The drawing under review shows one solid part. Ordinate dimensions are in mm from its lowest x, y, z. A direction names the side the tool comes from. Round coordinates to 2 decimals unless told otherwise and drop trailing zeros. Loops run counter-clockwise (first coordinate to the right, second up) from the corner with the lowest first, then second, coordinate; pieces in that order, holes last. Notation, with made-up numbers: (48.5, 16.25) -> (101.5, 16.25) arc R26 ccw to (101.5, 37.25) -> close; hole circle Ø4 at (-28, 15). An arc over 180 degrees is marked (long way). Use a Markdown table: item, result. Add a question column.
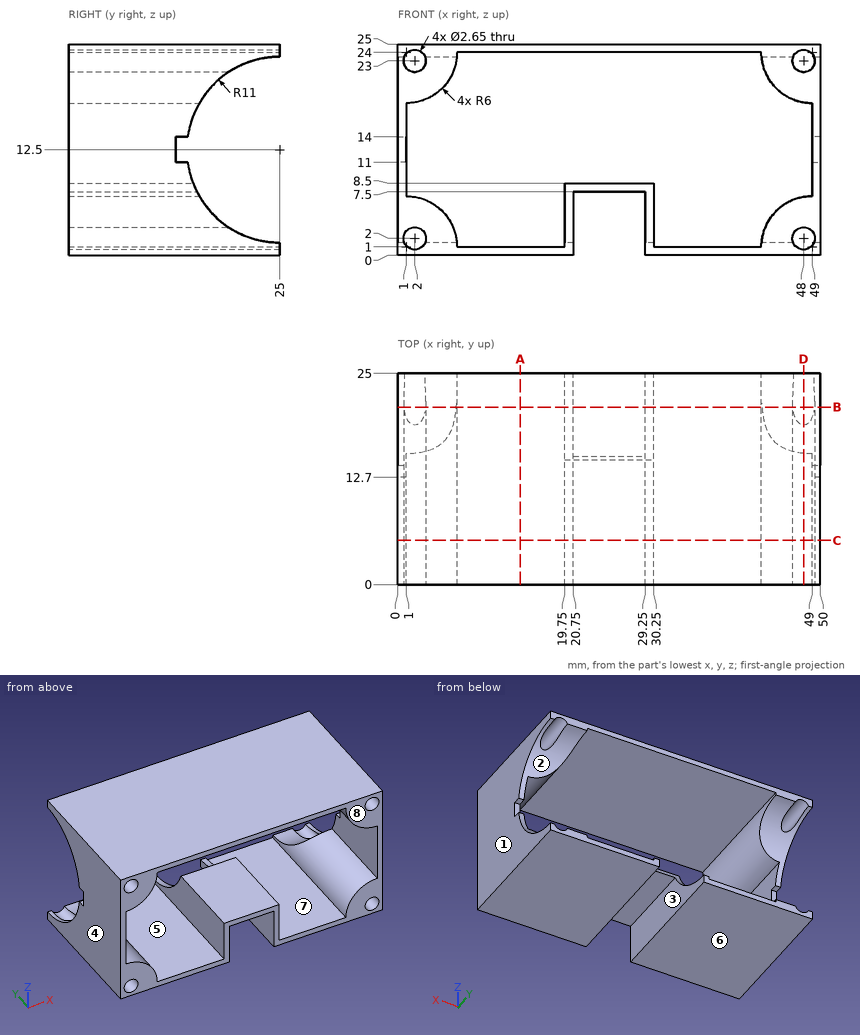
1. Consider section D-D on x = 48. State the section outline as (y, z) points (3 decimals).
2. To check wall thickness, follow probe 1 along Z at (x, y) = (40, 23.25); probe 2 along X at (y, z) = (1.75, 9.5); probe 3 along X at (y, z) = (2.25, 2) (3 decimals). State the ranges of each line that lie inside material, in increasing order. Write a range as from..to.
3. For the marked faces 1, 2, 3, 4 and 5, list the 3-axis set-ups (+Z, -Z, +X, -X, +Y, -Y) from which the entire face can be reached by the end or side of a thin tool; tool diameter is ignored.
4. Consider section B-B on y = 21. Give the number of separate pieces and of enclosed holes in the cut face, plus the area to 3 significant figures.
5. Insertion check: P1, Ø0.5, axis at x = 0.5, z = 12.5, coming from the +Y side; P2, Ø4, axis at x = 25.5, y = 6.5, coming from the -Z side. Each pin has a flat end and moves straight along its axis. Give the tip position at first contact, or say it passes through.
6. Consider section A-A on x = 14.5. State the section outline as (y, z) points, plus the area to 3 significant figures.
7. Consider section C-C on y = 5.25. State the section outline as (x, z) points (3 decimals).
8. Mouldability with a two-part tool opening along Z and no side actions: class the marked faces 6, 7 and 8 as +Z half, -Z half, draft (parallel to the pull), parting line (faces both ways), or undercut.
Verdict:
| question | item | result |
|---|---|---|
| 1 | outline | (0, 0) -> (25, 0) -> (25, 0.675) -> (0, 0.675) -> close; (0, 3.325) -> (18.932, 3.325) arc R11 cw to (15.523, 6.916) -> (0, 6.916) -> close; (0, 18.084) -> (15.523, 18.084) arc R11 cw to (18.932, 21.675) -> (0, 21.675) -> close; (0, 24.325) -> (25, 24.325) -> (25, 25) -> (0, 25) -> close |
| 2 | probe 1 | z = 0..1, 24..25 |
| 2 | probe 2 | x = 0..1, 49..50 |
| 2 | probe 3 | x = 0..0.675, 3.325..6.916, 19.75..20.75, 29.25..30.25, 43.084..46.675, 49.325..50 |
| 3 | face 1 | +Z, -Z, +X, +Y, -Y |
| 3 | face 2 | +X, -X, +Y |
| 3 | face 3 | -Z, +Y, -Y |
| 3 | face 4 | +Z, -Z, -X, +Y, -Y |
| 3 | face 5 | +Y, -Y |
| 4 | separate pieces | 3 |
| 4 | enclosed holes | 0 |
| 4 | area | 115 mm² |
| 5 | P1 | stops at y = 12.7 |
| 5 | P2 | stops at z = 7.5 |
| 6 | outline | (0, 0) -> (25, 0) -> (25, 1) -> (0, 1) -> close; (0, 24) -> (25, 24) -> (25, 25) -> (0, 25) -> close |
| 6 | area | 50.0 mm² |
| 7 | outline | (0, 0) -> (20.75, 0) -> (20.75, 7.5) -> (29.25, 7.5) -> (29.25, 0) -> (50, 0) -> (50, 25) -> (0, 25) -> close; hole circle Ø2.65 at (2, 2); hole circle Ø2.65 at (2, 23); hole (1, 7) arc R6 cw to (7, 1) -> (19.75, 1) -> (19.75, 8.5) -> (30.25, 8.5) -> (30.25, 1) -> (43, 1) arc R6 cw to (49, 7) -> (49, 18) arc R6 cw to (43, 24) -> (7, 24) arc R6 cw to (1, 18) -> close; hole circle Ø2.65 at (48, 2); hole circle Ø2.65 at (48, 23) |
| 8 | face 6 | -Z half |
| 8 | face 7 | undercut |
| 8 | face 8 | draft |
